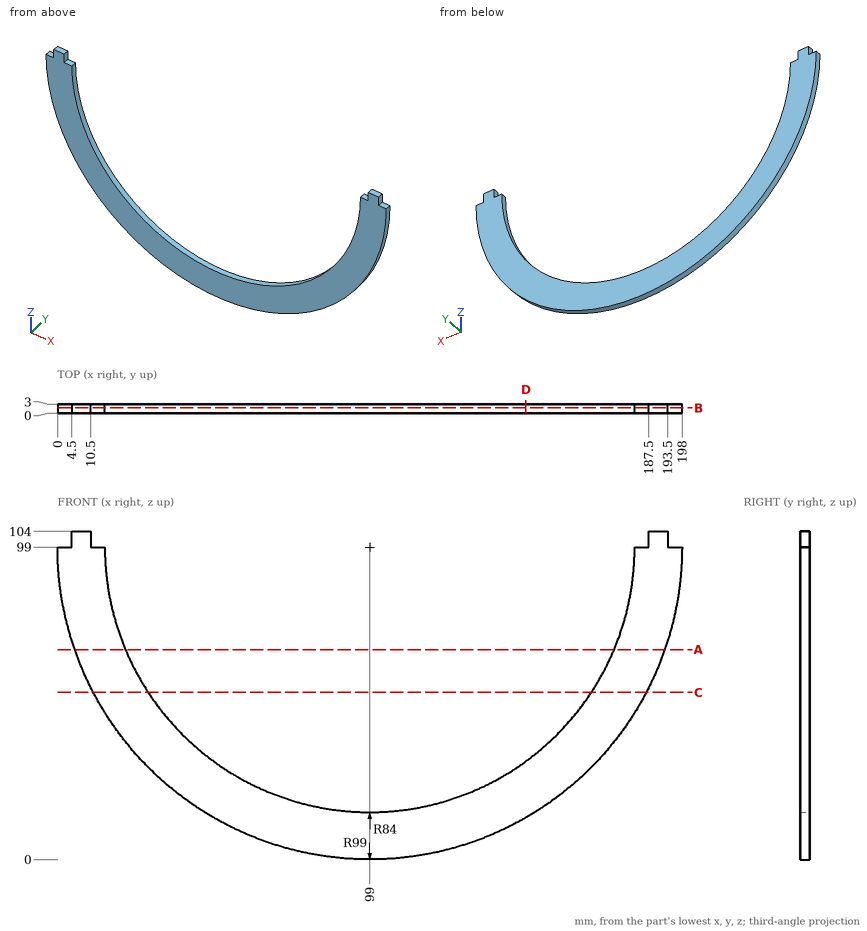
Design review of the part shown in the three views and the two pictorial views. Dimensions are in mm from the part's minimum x, y and z. Round coordinates to 2 decimals unless told otherwise and drop trailing zeros. Loops run counter-clockwise (first coordinate to the right, second up) from the corner with the lowest first, then second, coordinate; pieces in that order, holes last. Notation, with made-up numbers: M -31,-18 L 11,-18 A16 cw 11,13 Z; hole C 4,-31.5 d6. An arc over 180 degrees is marked long. Put each result on its own line as item: value.
Q1. Consider section A-A, the plane z = 66.5. Give the boundary of the cut face in (x, y), then the cut area to 3 significant figures.
Result set:
outline: M 5.49,0 L 21.54,0 L 21.54,3 L 5.49,3 Z; M 176.46,0 L 192.51,0 L 192.51,3 L 176.46,3 Z
area: 96.3 mm²
Q2. For pin 1 (4 mm diameter, centred on x = 173, z = 62.5, fed in from -Y); pin 2 (1 mm diameter, centred on x = 106.5, y = 1.5, fed in from -Z); pin 3 (1.5 mm diameter, centred on y = 1.5, z = 102, fed in from -X); pin 4 (1.5 mm diameter, centred on x = 186.5, y = 1, fed in from +Z), all flat-tipped, find the tip position at first contact; note any pin that passes through.
Result set:
pin 1: stops at y = 0
pin 2: stops at z = 0.25
pin 3: stops at x = 4.5
pin 4: stops at z = 99
Q3. Consider section D-D, the plane x = 148.5. Give the boundary of the cut face in (y, z), then the cut area to 3 significant figures.
Result set:
outline: M 0,13.26 L 3,13.26 L 3,31.13 L 0,31.13 Z
area: 53.6 mm²
Q4. To check wall thickness, follow L1, parallel to X at y = 2.85, z = 100.5; L2, parallel to X at y = 1.05, z = 56; L3, parallel to Z at x = 116.5, y = 2.8. State the ranges of each line that lie inside material, in increasing order.
Result set:
L1: x = 4.5 to 10.5, 187.5 to 193.5
L2: x = 9.83 to 26.84, 171.16 to 188.17
L3: z = 1.56 to 16.84
Q5. Consider section C-C, the plane z = 53. Give the boundary of the cut face in (x, y), then the cut area to 3 significant figures.
Result set:
outline: M 11.34,0 L 28.71,0 L 28.71,3 L 11.34,3 Z; M 169.29,0 L 186.66,0 L 186.66,3 L 169.29,3 Z
area: 104 mm²
Q6. Consider section B-B, the plane y = 1.75. Give the boundary of the cut face in (x, z), then the cut area to 3 significant figures.
Result set:
outline: M 0,99 A99 ccw 198,99 L 193.5,99 L 193.5,104 L 187.5,104 L 187.5,99 L 183,99 A84 cw 15,99 L 10.5,99 L 10.5,104 L 4.5,104 L 4.5,99 Z
area: 4,370 mm²
